Design review of the part built by this model. Coordinates are the model's own, in mm. Face numbers are marked on the shaded views. A direction names the side the tool comes from. Round coordinates to 2 decimals unless told otherwise and drop trailing zeros. Loops run counter-clockwise (first coordinate to the right, second up) from the corner with the lowest first, then second, coordinate; pieces in that order, holes last. Notation, with made-up numbers: (50.25, -13) - (77.25, -13) arc R16 ccw to (77.25, 3) - close; hole circle Ø10 at (11, 61.5). An arc over 180 degrees is marked (long way). One line per question, with ' | ' between items. Start each with the question number.
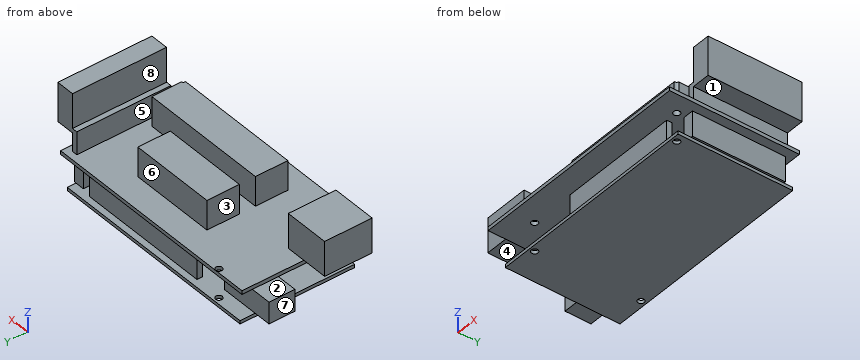
from build123d import *

# Parameters (mm, degrees)
ESBO_O1_W                 = 105
ESBO_O1_H                 = 60
RESSALTO_EXTRUS_O1_DEPTH  = 1.7
ESBO_O2_W                 = 60
ESBO_O2_H                 = 15
ESBO_O2_W_2               = 40
RESSALTO_EXTRUS_O2_DEPTH  = 13.6
RESSALTO_EXTRUS_O6_START  = 11.6
ESBO_O3_W                 = 100
ESBO_O3_H                 = 53
RESSALTO_EXTRUS_O6_DEPTH  = 1.5
ESBO_O4_W                 = 62.184169383
ESBO_O4_H                 = 2.54
ESBO_O4_W_2               = 5.08
ESBO_O4_H_2               = 42.957805244
ESBO_O4_W_3               = 56.07185462
RESSALTO_EXTRUS_O8_DEPTH  = 11.6
ESBO_O6_W                 = 21
ESBO_O6_H                 = 22
RESSALTO_EXTRUS_O9_DEPTH  = 16
ESBO_O7_W                 = 25.746964405
ESBO_O7_H                 = 12
RESSALTO_EXTRUS_O10_DEPTH = 10
ESBO_O8_R                 = 1.5
CORTE_EXTRUS_O1_DEPTH     = 78.869763066
RESSALTO_EXTRUS_O11_DEPTH = 56.905179102
CORTE_EXTRUS_O2_REACH     = 131.446


with BuildPart() as part:
    # Esbo_o1 → Ressalto-extrus_o1 (new body)
    with BuildSketch(Plane.XY):
        Rectangle(ESBO_O1_W, ESBO_O1_H)
    extrude(amount=RESSALTO_EXTRUS_O1_DEPTH)

    # Esbo_o2 → Ressalto-extrus_o2 (add)
    with BuildSketch(Plane.XY.offset(1.7)):
        with Locations((13.2, -12.2)):
            Rectangle(ESBO_O2_W, ESBO_O2_H)
        with Locations((3.2, 10.2)):
            Rectangle(ESBO_O2_W_2, ESBO_O2_H)
    extrude(amount=RESSALTO_EXTRUS_O2_DEPTH)



with BuildPart() as body_2:
    # Esbo_o3 → Ressalto-extrus_o6 (new body)
    with BuildSketch(Plane(origin=(0, 0, 0), x_dir=(-1, 0, 0), z_dir=(0, 0, -1)).offset(RESSALTO_EXTRUS_O6_START)):
        with Locations((2.5, 4.4)):
            Rectangle(ESBO_O3_W, ESBO_O3_H)
    extrude(amount=RESSALTO_EXTRUS_O6_DEPTH)


with BuildPart() as part_1:
    add(part.part)

    add(body_2.part)  # Ressalto-extrus_o8 merges body 2
    # Esbo_o4 → Ressalto-extrus_o8 (add)
    with BuildSketch(Plane.XY.offset(-11.6)):
        with Locations((7.150543675, 26.719832293)):
            Rectangle(ESBO_O4_W, ESBO_O4_H)
        with Locations((45.784919315, 5.42627648)):
            Rectangle(ESBO_O4_W_2, ESBO_O4_H_2)
        with Locations((10.206701056, -18.689881399)):
            Rectangle(ESBO_O4_W_3, ESBO_O4_H)
    extrude(amount=RESSALTO_EXTRUS_O8_DEPTH)

    # Esbo_o6 → Ressalto-extrus_o9 (add)
    with BuildSketch(Plane.XY.offset(1.7)):
        with Locations((-54, -9.6)):
            Rectangle(ESBO_O6_W, ESBO_O6_H)
    extrude(amount=RESSALTO_EXTRUS_O9_DEPTH)

    # Esbo_o7 → Ressalto-extrus_o10 (add)
    with BuildSketch(Plane.XY.offset(-11.6)):
        with Locations((-47.626517798, 17.9)):
            Rectangle(ESBO_O7_W, ESBO_O7_H)
    extrude(amount=RESSALTO_EXTRUS_O10_DEPTH)

    # Esbo_o8 → Corte-extrus_o1 (cut, through all)
    with BuildSketch(Plane(origin=(0, 0, -13.1), x_dir=(-1, 0, 0), z_dir=(0, 0, -1))):
        with Locations((37.26, 28.47)):
            Circle(ESBO_O8_R)
        with Locations((38.5, -19.7)):
            Circle(ESBO_O8_R)
        with Locations((-43.8, -19.7)):
            Circle(ESBO_O8_R)
    extrude(amount=-CORTE_EXTRUS_O1_DEPTH, mode=Mode.SUBTRACT)

    # Esbo_o9 → Ressalto-extrus_o11 (add)
    with BuildSketch(Plane.XZ.offset(30)):
        Polygon((49.5, 1.7), (49.5, 10.2), (58, 10.2), (58, 28.2), (49.5, 28.2), (49.5, 12.2), (47, 12.2), (47, 1.7), align=None)
    extrude(amount=-RESSALTO_EXTRUS_O11_DEPTH)

    # Corte-extrus_o2: up to this face of the body (flat: up to its plane)
    corte_extrus_o2_end = Plane(part_1.part.faces().sort_by_distance((47, -1.547410449, 6.95))[0])
    # Esbo_o10 → Corte-extrus_o2 (cut, up to the picked face)
    with BuildSketch(Plane(origin=(58, 0, 0), x_dir=(0, 0, -1), z_dir=(1, 0, 0)), mode=Mode.PRIVATE) as corte_extrus_o2_sk1:
        Polygon((-10.2, -16.57372352), (-28.2, -16.57372352), (-28.2, -30), (-1.7, -30), (-1.7, -16.57372352), align=None)
    corte_extrus_o2_tool1 = split(extrude(corte_extrus_o2_sk1.sketch, amount=-CORTE_EXTRUS_O2_REACH, mode=Mode.PRIVATE), bisect_by=corte_extrus_o2_end, keep=Keep.BOTH, mode=Mode.PRIVATE)
    add(corte_extrus_o2_tool1.solids().sort_by(Axis((58, -23.286862, 14.95), (-1, 0, 0)))[0], mode=Mode.SUBTRACT)


solid = part_1.part
1. Take a section at C-C, the plane y = -7. Give the boundary of the cut face in (x, z).
2. To check wall thickness, follow line 1 along Z through (x, y) = (8, 15.5); line 2 along Y through (x, z) = (-38.5, 0.85); line 3 along Z through (x, y) = (-8.5, -3.5). State the ranges of each line that lie inside material, in increasing order.
3. Take a section at B-B, the plane x = -30. Give the boundary of the cut face in (y, z).
4. Take a section at D-D, the plane z = -6.5. Give the boundary of the cut face in (x, y), then the cut area to 3 significant figures.
5. The part is to be moulded in two halves that separate along X. For the marked faces 5, 6, 7 and 8, say which applies: pulls with the +X half, pulls with the -X half, needs draft (parallel to the pull), parting line crosses it, or undercut.
6. Take a section at A-A, the plane z = 9. Give the boundary of the cut face in (x, y), then the cut area to 3 significant figures.
7. Clearance check with flat-ended pins moving along their axes: P1, Ø11, axis at x = -48.5, z = -7.5, coming from the -Y side; P2, Ø1, axis at y = 19.5, z = 4, coming from the +X side; P3, Ø4, axis at x = 17, y = -23.5, coming from the +Z side; P4, Ø2.5, axis at x = -38.5, y = -19.7, coming from the +Z side. State where each tip first meets the part, or that it passes through.
8. Machinability: for the marked faces 1, 2, 3 and 4, which of the approach directions +Z, -Z, +X, -X, +Y, -Y give a long, thin tool a straight path to every point of the face, cutting with its end or side? Answer none if there is none.
Answer list:
1) outline: (-64.5, 1.7) - (-52.5, 1.7) - (-52.5, 0) - (43.24, 0) - (43.24, -11.6) - (-52.5, -11.6) - (-52.5, -13.1) - (47.5, -13.1) - (47.5, -11.6) - (48.32, -11.6) - (48.32, 0) - (52.5, 0) - (52.5, 1.7) - (49.5, 1.7) - (49.5, 10.2) - (58, 10.2) - (58, 28.2) - (49.5, 28.2) - (49.5, 12.2) - (47, 12.2) - (47, 1.7) - (43.2, 1.7) - (43.2, 15.3) - (-16.8, 15.3) - (-16.8, 1.7) - (-43.5, 1.7) - (-43.5, 17.7) - (-64.5, 17.7) - close
2) line 1: z = -13.1 to -11.6, 0 to 15.3 | line 2: y = -30 to -21.2, -18.2 to 27.63, 29.31 to 30 | line 3: z = -13.1 to -11.6, 0 to 1.7
3) outline: (-30, 0) - (30, 0) - (30, 1.7) - (-30, 1.7) - close; (-22.1, -13.1) - (30.9, -13.1) - (30.9, -11.6) - (-22.1, -11.6) - close
4) outline: (-60.5, 11.9) - (-34.75, 11.9) - (-34.75, 23.9) - (-60.5, 23.9) - close; (-23.94, 25.45) - (38.24, 25.45) - (38.24, 27.99) - (-23.94, 27.99) - close; (-17.83, -19.96) - (38.24, -19.96) - (38.24, -17.42) - (-17.83, -17.42) - close; (43.24, -16.05) - (48.32, -16.05) - (48.32, 26.91) - (43.24, 26.91) - close | area: 828 mm²
5) face 5: undercut | face 6: needs draft | face 7: pulls with the -X half | face 8: undercut
6) outline: (-64.5, -20.6) - (-43.5, -20.6) - (-43.5, 1.4) - (-64.5, 1.4) - close; (-16.8, -19.7) - (42.3, -19.7) arc R1.5 cw to (43.2, -18.33) - (43.2, -4.7) - (-16.8, -4.7) - close; (-16.8, 2.7) - (23.2, 2.7) - (23.2, 17.7) - (-16.8, 17.7) - close; (47, -16.57) - (49.5, -16.57) - (49.5, 26.91) - (47, 26.91) - close | area: 2,070 mm²
7) P1: stops at y = -22.1 | P2: stops at x = 49.5 | P3: stops at z = 1.7 | P4: passes through
8) face 1: +X, +Y, -Y | face 2: -X, +Y, -Y | face 3: +Z, -X, +Y, -Y | face 4: -Z, -X, +Y, -Y
